Part model, mm, in its own coordinate system. A direction names the side the tool comes from. Give positions to 0.01 mm unless a question says otherwise; leave off trailing zeros. Write each loop counter-clockwise with the first axis right and the second up, starting at its lowest first coordinate (ties: lowest second). Pieces come first, ordered by that corner, then holes. Notation, with made-up numbers: M 35,-14.5 L 46,-14.5 A13 ccw 46,7.5 Z; hole C 56,-33.75 d9. An arc over 180 degrees is marked long. Answer as CSV lines item,"result". Start each with the question number.
Item 1: Band-saw the part on B-B, the plane y = 0. List the corners of the cut face in (x, z).
Item 2: Two-plate mould, pull along Y, no slides. Class faces 1 (the flat face through (174.7, 20.264, 0.5)), 2 (the flat face through (175.4, -20.264, 0.5)), 3 (the flat face through (173.14, 5.49, 1.54)): +Y half, -Y half, draft (parallel to the pull), parting line (faces both ways), or undercut.
Item 3: Band-saw the part on C-C, the plane x = 180.5. List the corners of the cut face in (y, z), then the cut area to 3 significant figures.
Item 4: 3-axis set-ups, long thin cutter, end or side, ignore diameter. For faces 4 (the cylindrical face through (196.5, 0.3, 0.5)), 5 (the flat face through (173.1, 5, 0.5)), 6 (the conical face through (187.42, 0.11, 1.24)): which of +Z, -Z, +X, -X, +Y, -Y reach the whole face in a straight line?
Item 5: Wall check: L1, parallel to Y at x = 152, z = 0.8; L2, parallel to Y at x = 153.5, z = 1.7; L3, parallel to Y at x = 167, z = 0.85. Give the ranges that are in metal, low to high. Write a range as from..to.
Item 6: Band-saw the part on A-A, the plane x = 172. List the corners of the cut face in (y, z).
from build123d import *
from OCP.BRepFilletAPI import BRepFilletAPI_MakeChamfer

# Parameters (mm, degrees)
SKETCH_2_R      = 1.45
EXTRUDE_1_DEPTH = 2
CHAMFER_2_SIZE  = 1
CHAMFER_2_SIZE2 = 0.900404044
CHAMFER_3_SIZE  = 1
CHAMFER_3_SIZE2 = 0.900404044


with BuildPart() as part:
    # 草图2 → 凸台-拉伸1 (new body)
    with BuildSketch(Plane.XY):
        with BuildLine():
            Line((148.264880132, -17.264045876), (148.264880132, 17.264045876))
            ThreePointArc((148.264880132, 17.264045876), (149.143559788, 19.385366219), (151.264880132, 20.264045876))
            Line((151.264880132, 20.264045876), (198.85204531, 20.264045876))
            ThreePointArc((198.85204531, 20.264045876), (200.555549989, 19.311935091), (200.637129492, 17.362117684))
            ThreePointArc((200.637129492, 17.362117684), (196.5, 0), (200.637129492, -17.362117684))
            ThreePointArc((200.637129492, -17.362117684), (200.555549989, -19.311935091), (198.85204531, -20.264045876))
            Line((198.85204531, -20.264045876), (151.264880132, -20.264045876))
            ThreePointArc((151.264880132, -20.264045876), (149.143559788, -19.385366219), (148.264880132, -17.264045876))
        make_face()
        with Locations((152.264880132, 16.264045876)):
            Circle(SKETCH_2_R, mode=Mode.SUBTRACT)
        with Locations((181.264880132, 16.264045876)):
            Circle(SKETCH_2_R, mode=Mode.SUBTRACT)
        with Locations((195.735119868, 16.264045876)):
            Circle(SKETCH_2_R, mode=Mode.SUBTRACT)
        with Locations((152.264880132, -16.264045876)):
            Circle(SKETCH_2_R, mode=Mode.SUBTRACT)
        with Locations((181.264880132, -16.264045876)):
            Circle(SKETCH_2_R, mode=Mode.SUBTRACT)
        with Locations((195.735119868, -16.264045876)):
            Circle(SKETCH_2_R, mode=Mode.SUBTRACT)
        with BuildLine():
            Line((164.264880132, 5), (182.264880132, 5))
            ThreePointArc((182.264880132, 5), (187.264880132, 0), (182.264880132, -5))
            Line((182.264880132, -5), (164.264880132, -5))
            ThreePointArc((164.264880132, -5), (159.264880132, 0), (164.264880132, 5))
        make_face(mode=Mode.SUBTRACT)
    extrude(amount=EXTRUDE_1_DEPTH)

    # 倒角2: one chamfer whose edges measure the first distance from different faces: ONE call of the kernel's chamfer builder (chamfer() names one face for all edges)
    chamfer_2_edges_1 = [part.edges().sort_by_distance(p)[0] for p in [
        (200.555549989, -19.311935091, 2),
    ]]
    chamfer_2_side_1 = [part.faces().sort_by_distance(p)[0] for p in [
        (200.555549989, -19.311935091, 1),
    ]]
    chamfer_2_edges_2 = [part.edges().sort_by_distance(p)[0] for p in [
        (196.5, 0, 2),
    ]]
    chamfer_2_side_2 = [part.faces().sort_by_distance(p)[0] for p in [
        (196.5, 0, 1),
    ]]
    chamfer_2_edges_3 = [part.edges().sort_by_distance(p)[0] for p in [
        (200.555549989, 19.311935091, 2),
    ]]
    chamfer_2_side_3 = [part.faces().sort_by_distance(p)[0] for p in [
        (200.555549989, 19.311935091, 1),
    ]]
    chamfer_2_edges_4 = [part.edges().sort_by_distance(p)[0] for p in [
        (175.058462721, 20.264045876, 2),
    ]]
    chamfer_2_side_4 = [part.faces().sort_by_distance(p)[0] for p in [
        (175.058462721, 20.264045876, 1),
    ]]
    chamfer_2_edges_5 = [part.edges().sort_by_distance(p)[0] for p in [
        (149.143559788, 19.385366219, 2),
    ]]
    chamfer_2_side_5 = [part.faces().sort_by_distance(p)[0] for p in [
        (149.143559788, 19.385366219, 1),
    ]]
    chamfer_2_edges_6 = [part.edges().sort_by_distance(p)[0] for p in [
        (148.264880132, 0, 2),
    ]]
    chamfer_2_side_6 = [part.faces().sort_by_distance(p)[0] for p in [
        (148.264880132, 0, 1),
    ]]
    chamfer_2_edges_7 = [part.edges().sort_by_distance(p)[0] for p in [
        (149.143559788, -19.385366219, 2),
    ]]
    chamfer_2_side_7 = [part.faces().sort_by_distance(p)[0] for p in [
        (149.143559788, -19.385366219, 1),
    ]]
    chamfer_2_edges_8 = [part.edges().sort_by_distance(p)[0] for p in [
        (175.058462721, -20.264045876, 2),
    ]]
    chamfer_2_side_8 = [part.faces().sort_by_distance(p)[0] for p in [
        (175.058462721, -20.264045876, 1),
    ]]
    chamfer_2 = BRepFilletAPI_MakeChamfer(part.part.solid().wrapped)
    for e in chamfer_2_edges_1:
        chamfer_2.Add(CHAMFER_2_SIZE, CHAMFER_2_SIZE2, e.wrapped, chamfer_2_side_1[0].wrapped)  # the first distance lies on this face
    for e in chamfer_2_edges_2:
        chamfer_2.Add(CHAMFER_2_SIZE, CHAMFER_2_SIZE2, e.wrapped, chamfer_2_side_2[0].wrapped)  # the first distance lies on this face
    for e in chamfer_2_edges_3:
        chamfer_2.Add(CHAMFER_2_SIZE, CHAMFER_2_SIZE2, e.wrapped, chamfer_2_side_3[0].wrapped)  # the first distance lies on this face
    for e in chamfer_2_edges_4:
        chamfer_2.Add(CHAMFER_2_SIZE, CHAMFER_2_SIZE2, e.wrapped, chamfer_2_side_4[0].wrapped)  # the first distance lies on this face
    for e in chamfer_2_edges_5:
        chamfer_2.Add(CHAMFER_2_SIZE, CHAMFER_2_SIZE2, e.wrapped, chamfer_2_side_5[0].wrapped)  # the first distance lies on this face
    for e in chamfer_2_edges_6:
        chamfer_2.Add(CHAMFER_2_SIZE, CHAMFER_2_SIZE2, e.wrapped, chamfer_2_side_6[0].wrapped)  # the first distance lies on this face
    for e in chamfer_2_edges_7:
        chamfer_2.Add(CHAMFER_2_SIZE, CHAMFER_2_SIZE2, e.wrapped, chamfer_2_side_7[0].wrapped)  # the first distance lies on this face
    for e in chamfer_2_edges_8:
        chamfer_2.Add(CHAMFER_2_SIZE, CHAMFER_2_SIZE2, e.wrapped, chamfer_2_side_8[0].wrapped)  # the first distance lies on this face
    add(Compound.cast(chamfer_2.Shape()), mode=Mode.REPLACE)

    # 倒角3
    chamfer_3_edges = [part.edges().sort_by_distance(p)[0] for p in [
        (159.264880132, 0, 2),
        (173.264880132, -5, 2),
        (187.264880132, 0, 2),
        (173.264880132, 5, 2),
    ]]
    chamfer_3_side = [part.faces().sort_by_distance(p)[0] for p in [
        (199.244635879, -18.505542966, 2),
    ]]
    chamfer(chamfer_3_edges, length=CHAMFER_3_SIZE, length2=CHAMFER_3_SIZE2, reference=chamfer_3_side[0])


solid = part.part
Output:
1,outline,"M 148.26,0 L 159.26,0 L 159.26,1.1 L 158.26,2 L 149.17,2 L 148.26,1 Z; M 187.26,0 L 196.5,0 L 196.5,1 L 195.6,2 L 188.26,2 L 187.26,1.1 Z"
2,face 1,"+Y half"
2,face 2,"-Y half"
2,face 3,"undercut"
3,outline,"M -20.26,0 L -17.5,0 L -17.5,2 L -19.36,2 L -20.26,1 Z; M -15.03,0 L -5,0 L -5,1.1 L -6,2 L -15.03,2 Z; M 5,0 L 15.03,0 L 15.03,2 L 6,2 L 5,1.1 Z; M 17.5,0 L 20.26,0 L 20.26,1 L 19.36,2 L 17.5,2 Z"
3,area,"49.4 mm²"
4,face 4,"+Z, -Z, +X"
4,face 5,"+Z, -Z"
4,face 6,"+Z"
5,L1,"-20.26..-17.69, -14.84..14.84, 17.69..20.26"
5,L2,"-19.63..-17.02, -15.5..15.5, 17.02..19.63"
5,L3,"-20.26..-5, 5..20.26"
6,outline,"M -20.26,0 L -5,0 L -5,1.1 L -6,2 L -19.36,2 L -20.26,1 Z; M 5,0 L 20.26,0 L 20.26,1 L 19.36,2 L 6,2 L 5,1.1 Z"
